Design review of the part built by this model. Coordinates are the model's own, in mm. Coordinates: 2 decimals unless noted, no trailing zeros. Write item = value, one per line.
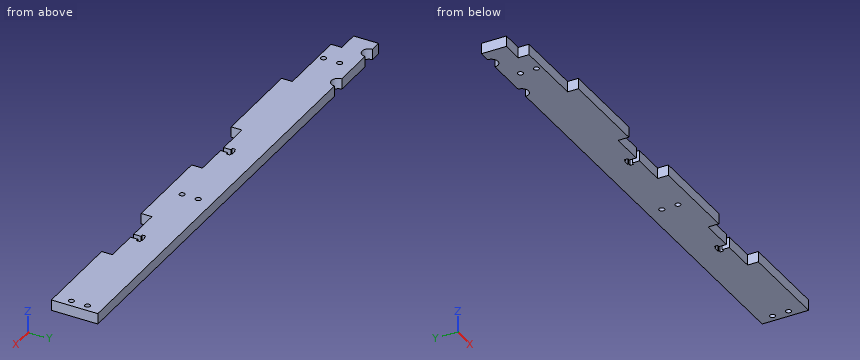
```python
from build123d import *

# Parameters (mm, degrees)
SZKIC1_W                    = 284
SZKIC1_H                    = 26
DODANIE_WYCI_GNI_CIE1_DEPTH = 6
SZKIC5_W                    = 40
SZKIC5_H                    = 6
WYTNIJ_WYCI_GNI_CIE3_DEPTH  = 6
SZYK_LINIOWY1_COUNT         = 4
SZYK_LINIOWY1_PITCH         = 91
WYTNIJ_WYCI_GNI_CIE4_DEPTH  = 6
SZYK_LINIOWY2_COUNT         = 2
SZYK_LINIOWY2_PITCH         = 91
SZKIC9_W                    = 12
SZKIC9_H                    = 12
WYTNIJ_WYCI_GNI_CIE6_DEPTH  = 10
SZKIC10_R                   = 1.5
WYTNIJ_WYCI_GNI_CIE7_DEPTH  = 10
SZKIC12_R                   = 3.75
WYTNIJ_WYCI_GNI_CIE8_DEPTH  = 6


with BuildPart() as part:
    # Szkic1 → Dodanie-wyciągnięcie1 (new body)
    with BuildSketch(Plane.XY):
        with Locations((-737.9, 7)):
            Rectangle(SZKIC1_W, SZKIC1_H)
    extrude(amount=-DODANIE_WYCI_GNI_CIE1_DEPTH)

    # Szkic5 → Wytnij-wyciągnięcie3 (cut)
    with BuildSketch(Plane.XY):
        with Locations((-666.76, -3)):
            Rectangle(SZKIC5_W, SZKIC5_H)
    wytnij_wyci_gni_cie3 = extrude(amount=-WYTNIJ_WYCI_GNI_CIE3_DEPTH, mode=Mode.SUBTRACT)

    # Szyk liniowy1: Wytnij-wyciągnięcie3 ×4
    with Locations(*[(-i * SZYK_LINIOWY1_PITCH, 0, 0) for i in range(1, SZYK_LINIOWY1_COUNT)]):
        add(wytnij_wyci_gni_cie3, mode=Mode.SUBTRACT)

    # Szkic6 → Wytnij-wyciągnięcie4 (cut)
    with BuildSketch(Plane.XY):
        Polygon((-665.21, 0), (-668.31, 0), (-668.31, 4), (-669.685, 4), (-669.685, 6), (-668.31, 6), (-668.31, 6.5), (-665.21, 6.5), (-665.21, 6), (-663.835, 6), (-663.835, 4), (-665.21, 4), align=None)
    wytnij_wyci_gni_cie4 = extrude(amount=-WYTNIJ_WYCI_GNI_CIE4_DEPTH, mode=Mode.SUBTRACT)

    # Szyk liniowy2: Wytnij-wyciągnięcie4 ×2
    with Locations(*[(-i * SZYK_LINIOWY2_PITCH, 0, 0) for i in range(1, SZYK_LINIOWY2_COUNT)]):
        add(wytnij_wyci_gni_cie4, mode=Mode.SUBTRACT)

    # Szkic9 → Wytnij-wyciągnięcie6 (cut)
    with BuildSketch(Plane.XY):
        with Locations((-873.9, 0)):
            Rectangle(SZKIC9_W, SZKIC9_H)
    extrude(amount=-WYTNIJ_WYCI_GNI_CIE6_DEPTH, mode=Mode.SUBTRACT)

    # Szkic10 → Wytnij-wyciągnięcie7 (cut)
    with BuildSketch(Plane.XY):
        with Locations((-599.9, 3)):
            Circle(SZKIC10_R)
        with Locations((-599.9, 12)):
            Circle(SZKIC10_R)
        with Locations((-854.9, 3)):
            Circle(SZKIC10_R)
        with Locations((-854.9, 12)):
            Circle(SZKIC10_R)
        with Locations((-711.9, 3)):
            Circle(SZKIC10_R)
        with Locations((-711.9, 12)):
            Circle(SZKIC10_R)
    extrude(amount=-WYTNIJ_WYCI_GNI_CIE7_DEPTH, mode=Mode.SUBTRACT)

    # Szkic12 → Wytnij-wyciągnięcie8 (cut)
    with BuildSketch(Plane.XY):
        with Locations((-838.918997424, 20.044165404)):
            Circle(SZKIC12_R)
        with Locations((-869.918997424, 20.044165404)):
            Circle(SZKIC12_R)
    extrude(amount=-WYTNIJ_WYCI_GNI_CIE8_DEPTH, mode=Mode.SUBTRACT)


solid = part.part
```
Q1. Wall thickness on line 1 (Y direction, x = -711.9, z = -3.9); line 2 (X direction, y = -0.75, z = -4.55); line 3 (Y direction, x = -854.9, z = -2.9): over which ranges is each line inside the solid? List them lowest first.
Check result:
line_1 = -6 to 1.5, 4.5 to 10.5, 13.5 to 20
line_2 = -828.76 to -777.76, -737.76 to -686.76, -646.76 to -595.9
line_3 = 0 to 1.5, 4.5 to 10.5, 13.5 to 20
Q2. Consider section A-A, the plane z = -3.6. State how many separate pieces and enclosed holes the cut face has, and give its area (3 significant figures).
Check result:
separate_pieces = 1
enclosed_holes = 6
area = 6,390 mm²
Q3. For P1, Ø0.9, axis at x = -666.5, z = -3.5, coming from the -Y side; P2, Ø1, axis at x = -836.5, z = -2, coming from the +Y side; P3, Ø1.8, axis at y = -4.5, z = -2.5, coming from the -X side, all flat-tipped, find the tip position at first contact; note any pin that passes through.
Check result:
P1 = 6.5
P2 = 17.69
P3 = -828.76
